```python
from build123d import *

# Parameters (mm, degrees)
EXTRUDE_START          = 1.25
EXTRUDE_1_DEPTH        = 2.5
SKETCH_2_R             = 7.5
CUT_EXTRUDE_1_DEPTH    = 32.659095027
PATTERN_LINEAR_1_COUNT = 2
PATTERN_LINEAR_1_PITCH = 80.45
SKETCH_3_W             = 52.302227504
SKETCH_3_H             = 11.68512329
EXTRUDE_2_DEPTH        = 5
FILLET_1_R             = 10
SKETCH_4_R             = 1.5
CUT_EXTRUDE_2_DEPTH    = 103.123184877
SKETCH_5_R             = 1.5
CUT_EXTRUDE_3_DEPTH    = 103.123184877


with BuildPart() as part:
    # Sketch 1 → Extrude 1 (new, symmetric)
    with BuildSketch(Plane.XY.offset(EXTRUDE_START)):
        with BuildLine():
            Line((-18.36323223, 0), (18.36323223, 0))
            Line((18.36323223, 0), (12.203770764, 16.779729806))
            ThreePointArc((12.203770764, 16.779729806), (0, 25.3), (-12.203770764, 16.779729806))
            Line((-12.203770764, 16.779729806), (-18.36323223, 0))
        make_face()
    extrude(amount=EXTRUDE_1_DEPTH, both=True)

    # Sketch 2 → Cut-Extrude 1 (cut, through all)
    with BuildSketch(Plane.XY.offset(3.75)):
        with Locations((0, 12.3)):
            Circle(SKETCH_2_R)
    extrude(amount=-CUT_EXTRUDE_1_DEPTH, mode=Mode.SUBTRACT)


with BuildPart() as pattern_linear_1_1:
    # Pattern Linear 1: pattern copy
    add(part.part.moved(Location(Vector(1, 0, 0) * (1 * PATTERN_LINEAR_1_PITCH))))


with BuildPart() as part_1:
    add(part.part)

    add(pattern_linear_1_1.part)  # Extrude 2 merges Pattern Linear 1_1
    # Sketch 3 → Extrude 2 (add)
    with BuildSketch(Plane(origin=(0, 0, -1.25), x_dir=(-1, 0, 0), z_dir=(0, 0, -1))):
        with Locations((-40.225, 5.842561645)):
            Rectangle(SKETCH_3_W, SKETCH_3_H)
    extrude(amount=-EXTRUDE_2_DEPTH)

    # Fillet 1
    fillet_1_edges = [part_1.edges().sort_by_distance(p)[0] for p in [
        (14.073886248, 11.68512329, 1.25),
        (66.376113752, 11.68512329, 1.25),
    ]]
    fillet(fillet_1_edges, radius=FILLET_1_R)

    # Sketch 4 → Cut-Extrude 2 (cut, through all)
    with BuildSketch(Plane(origin=(0, 0, -1.25), x_dir=(-1, 0, 0), z_dir=(0, 0, -1))):
        with Locations((1.598414444, 21.66456466)):
            Circle(SKETCH_4_R)
        with Locations((7.310743669, 6.233450156)):
            Circle(SKETCH_4_R)
        with Locations((-8.909158113, 9.001985185)):
            Circle(SKETCH_4_R)
        with Locations((-71.540841887, 15.598014815)):
            Circle(SKETCH_4_R)
        with Locations((-82.048414444, 2.93543534)):
            Circle(SKETCH_4_R)
        with Locations((-87.760743669, 18.366549844)):
            Circle(SKETCH_4_R)
    extrude(amount=-CUT_EXTRUDE_2_DEPTH, mode=Mode.SUBTRACT)

    # Sketch 5 → Cut-Extrude 3 (cut, through all)
    with BuildSketch(Plane(origin=(0, 0, -1.25), x_dir=(-1, 0, 0), z_dir=(0, 0, -1))):
        with Locations((-93.225, 4)):
            Circle(SKETCH_5_R)
        with Locations((-53.225, 4)):
            Circle(SKETCH_5_R)
        with Locations(Location((12.775, 4, 0), (0, 0, 180))):
            Circle(SKETCH_5_R)
        with Locations(Location((-27.225, 4, 0), (0, 0, 180))):
            Circle(SKETCH_5_R)
    extrude(amount=-CUT_EXTRUDE_3_DEPTH, mode=Mode.SUBTRACT)


solid = part_1.part
```
Check sheet for the modelled part. Datum: model origin and axes. Units: mm. Give positions to 0.01 mm unless a question says otherwise; leave off trailing zeros. Order: outer loops, then holes, each group sorted by start corner. A loop starts at its lowest first (then second) coordinate and runs counter-clockwise, first axis right, second up. Notation, with made-up numbers: (-13.75, -36) -> (40.25, -36) arc R13 cw to (40.25, -12) -> close; hole circle Ø5 at (56, 80). An arc over 180 degrees is marked (long way). Return JSON: item names as keys, results as strings.
1. Material ranges on probe 1 along X at (y, z) = (4.5, 2.2); probe 2 along X at (y, z) = (16.5, 1.6); probe 3 along Y at (x, z) = (-6, -0.35), recorded low to high. Write a range as [from, to].
From the geometry:
{"probe 1": "[-16.71, -14.19], [-11.36, 25.81], [28.64, 51.81], [54.64, 91.81], [94.64, 97.16]", "probe 2": "[-12.31, -6.21], [6.21, 12.45], [68, 70.34], [72.74, 74.24], [86.66, 92.76]", "probe 3": "[0, 5.5], [6.96, 7.8], [16.8, 23.83]"}
2. Mould release check, pull along Y, two halves, no side actions. Record for faces 1 (the flat face through (39, 0, 1)), 2 (the cylindrical face through (-1.63, 4.98, 1.28)), 3 (the cylindrical face through (81.24, 4.2, 1.21)), 4 (the flat face through (95.777, 8.272, 1.285)): +Y half, -Y half, draft (parallel to the pull), parting line (faces both ways), or undercut.
From the geometry:
{"face 1": "-Y half", "face 2": "undercut", "face 3": "undercut", "face 4": "+Y half"}
3. Cross-section at A-A, the plane x = 57. Record the cut outline in (y, z).
From the geometry:
{"outline": "(0, -1.25) -> (11.69, -1.25) -> (11.69, 3.75) -> (0, 3.75) -> close"}
4. Go/stop test with flat-tipped pins: P1, Ø2, axis at y = 9.5, z = 0, coming from the -X side; P2, Ø3, axis at x = 48, z = -0.5, coming from the +Y side. Record where each tip stops, or that it passes through.
From the geometry:
{"P1": "x = -15.24", "P2": "y = 11.69"}
5. Cross-section at B-B, the plane z = 1.85. Count the separate pieces of the cut face and the enclosed holes in it, plus the area to 3 significant figures.
From the geometry:
{"separate pieces": "1", "enclosed holes": "12", "area": "1,480 mm^2"}
